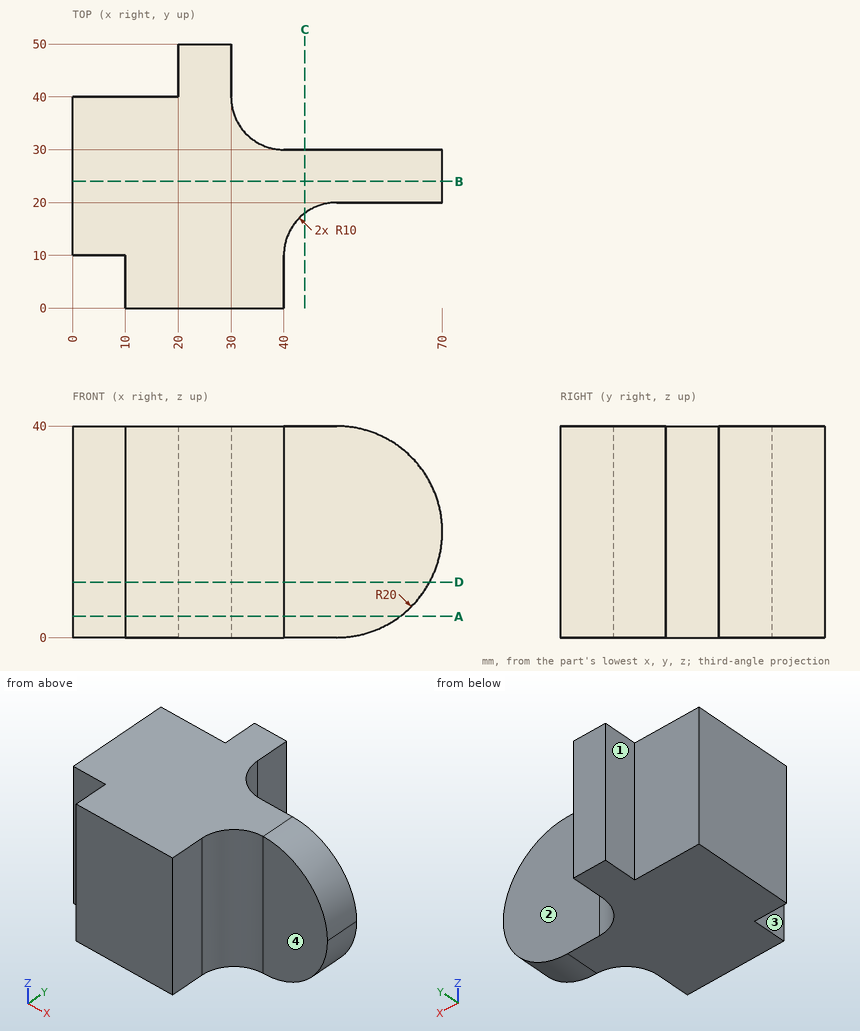
Could you check a few things on this drawing? It's one solid part, dimensions in mm from its lowest x, y, z. A direction names the side the tool comes from. Give positions to 0.01 mm unless a question says otherwise; leave off trailing zeros. Order: outer loops, then holes, each group sorted by start corner. A loop starts at its lowest first (then second) coordinate and runs counter-clockwise, first axis right, second up.
1. Suppose I cut it at A-A (z = 4). Write out the boundary of the cut face in (x, y).
Answers below:
outline: (0, 10) - (10, 10) - (10, 0) - (40, 0) - (40, 10) arc R10 cw to (50, 20) - (62, 20) - (62, 30) - (40, 30) arc R10 cw to (30, 40) - (30, 50) - (20, 50) - (20, 40) - (0, 40) - close
2. For pin 1 (10 mm diameter, centred on x = 57, z = 16.5, fed in from -Y); pin 2 (3 mm diameter, centred on y = 45.5, z = 13, fed in from -X); pin 3 (6 mm diameter, centred on x = 8.5, z = 13, fed in from +Y), each with a flat end and sliding along its axis, tell me the tip position at first contact or that it passes through.
Answers below:
pin 1: stops at y = 20
pin 2: stops at x = 20
pin 3: stops at y = 40
3. I need wall thicknesses on L1, parallel to Y at x = 19, z = 28.5; L2, parallel to X at y = 47, z = 16. Which ranges of each line are inside material? Lowest first, please.
Answers below:
L1: y = 0 to 40
L2: x = 20 to 30
4. Which directions (+Z, -Z, +X, -X, +Y, -Y) give clear straight access to the entire face, cutting with the end or side of a thin tool? Please do the marked faces 1, 2, 3 and 4.
Answers below:
face 1: +Z, -Z, -X, +Y
face 2: +Z, -Z, +X, +Y
face 3: +Z, -Z, -X, -Y
face 4: +Z, -Z, +X, -Y
5. Suppose I cut it at B-B (y = 24). Write out the boundary of the cut face in (x, z).
Answers below:
outline: (0, 0) - (50, 0) arc R20 ccw to (50, 40) - (0, 40) - close
6. Suppose I cut it at D-D (z = 10.5). Write out the boundary of the cut face in (x, y), plus the area to 3 significant figures.
Answers below:
outline: (0, 10) - (10, 10) - (10, 0) - (40, 0) - (40, 10) arc R10 cw to (50, 20) - (67.6, 20) - (67.6, 30) - (40, 30) arc R10 cw to (30, 40) - (30, 50) - (20, 50) - (20, 40) - (0, 40) - close
area: 1,820 mm2
7. Suppose I cut it at C-C (x = 44). Write out the boundary of the cut face in (y, z), plus the area to 3 significant figures.
Answers below:
outline: (18, 0) - (30, 0) - (30, 40) - (18, 40) - close
area: 480 mm2
